The listing builds one solid part. Answer for the finished solid, in the listing's coordinates (mm). Face numbers are marked on the shaded views. A direction names the side the tool comes from. Coordinates: 2 decimals unless noted, no trailing zeros. Loops run counter-clockwise (first coordinate to the right, second up) from the corner with the lowest first, then second, coordinate; pieces in that order, holes last. Notation, with made-up numbers: (6, 72) - (13, 72) arc R18 cw to (13, 96) - close; hole circle Ø1 at (63.5, 28.5). An arc over 180 degrees is marked (long way). Write each question's results on one line, items separated by ' | '. Start each with the question number.
(1) Find section B-B on y = 14.5. Determine the outline of the cut face in (x, z) (3 decimals).
(2) Find section C-C on z = -31. Determine the outline of the cut face in (x, y) (3 decimals).
(3) For the marked faces 1 and 2, determine the directions among +Z, -Z, +X, -X, +Y, -Y from which every point of the face is accessible in a straight line to the end or side of a thin tool.
(4) Given pin 1 Ø1 at (x, y) = (-14.5, 12) entering from +Z; pin 2 Ø1.5 at (x, z) = (34.5, 5.5) entering from +Y (3 decimals); pin 3 Ø0.8 at (x, y) = (49, 13) entering from +Z (3 decimals); pin 4 Ø4.5 at (x, z) = (47.625, 57.15) entering from -Y, each flat-ended and moving along its own axis, determine where each tip first touches the part or whether it passes through.
(5) Determine the mould class of the marked faces 3, 4 and 5 for opening direction X: released by +X, released by -X, zero draft, split by the parting line, or undercut.
(6) Find section D-D on x = -26.5. Determine the outline of the cut face in (y, z) (3 decimals).
(7) Find section A-A on z = 57.15. Determine the outline of the cut face in (x, y) (3 decimals), then the cut area to 3 significant figures.
(8) Consider line 1 (X direction, y = 1.9, z = 44.45); line 2 (X direction, y = 14.75, z = 38.5); line 3 (Z direction, x = -16, y = 20.5). Determine where each line is inside the solid, lowest interval first. Write a range as from..to.
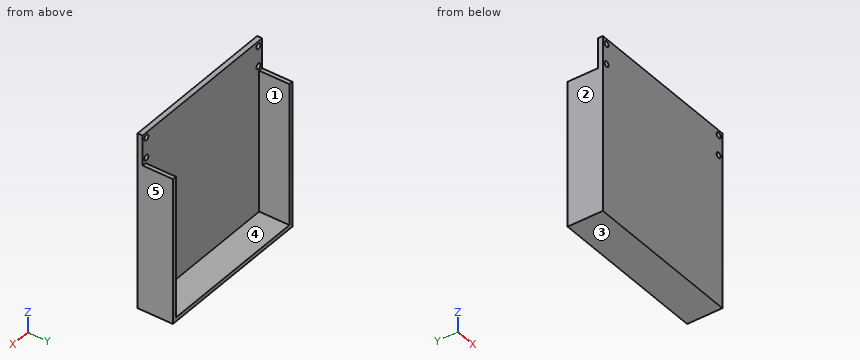
from build123d import *

# Parameters (mm, degrees)
SKETCH1_W             = 101.6
SKETCH1_H             = 101.6
SKETCH1_W_2           = 6.35
SKETCH1_H_2           = 9.525
BOSS_EXTRUDE1_DEPTH   = 3.175
F_8_32_TAPPED_HOLE1_D = 3.4544
BOSS_EXTRUDE2_DEPTH   = 19.05
SKETCH1_3_W           = 88.9
SKETCH1_3_H           = 9.525
BOSS_EXTRUDE3_DEPTH   = 3.175


with BuildPart() as part:
    # Sketch1 → Boss-Extrude1 (new body)
    with BuildSketch(Plane(origin=(0, 0, 0), x_dir=(1, 0, 0), z_dir=(0, 1, 0))):
        Rectangle(SKETCH1_W, SKETCH1_H)
        with Locations((-47.625, -55.5625)):
            Rectangle(SKETCH1_W_2, SKETCH1_H_2)
        with Locations((47.625, -55.5625)):
            Rectangle(SKETCH1_W_2, SKETCH1_H_2)
    extrude(amount=BOSS_EXTRUDE1_DEPTH)

    # #8-32 Tapped Hole1 (through all)
    with Locations(Plane(origin=(0, 0, 0), x_dir=(-1, 0, 0), z_dir=(0, -1, 0))):
        with Locations((-47.625, -57.15), (-47.625, -44.45), (47.625, -57.15), (47.625, -44.45)):
            Hole(F_8_32_TAPPED_HOLE1_D / 2)

    # Sketch8 → Boss-Extrude2 (add)
    with BuildSketch(Plane(origin=(0, 3.175, 0), x_dir=(1, 0, 0), z_dir=(0, 1, 0))):
        Polygon((-50.8, 50.8), (50.8, 50.8), (50.8, -41.275), (48.26, -41.275), (48.26, 48.26), (-48.26, 48.26), (-48.26, -41.275), (-50.8, -41.275), align=None)
    extrude(amount=BOSS_EXTRUDE2_DEPTH)

    # Sketch1<3> → Boss-Extrude3 (add)
    with BuildSketch(Plane(origin=(0, 0, 0), x_dir=(1, 0, 0), z_dir=(0, 1, 0))):
        with Locations((0, -55.5625)):
            Rectangle(SKETCH1_3_W, SKETCH1_3_H)
    extrude(amount=BOSS_EXTRUDE3_DEPTH)


solid = part.part
Values:
1) outline: (-50.8, -50.8) - (50.8, -50.8) - (50.8, 41.275) - (48.26, 41.275) - (48.26, -48.26) - (-48.26, -48.26) - (-48.26, 41.275) - (-50.8, 41.275) - close
2) outline: (-50.8, 0) - (50.8, 0) - (50.8, 22.225) - (48.26, 22.225) - (48.26, 3.175) - (-48.26, 3.175) - (-48.26, 22.225) - (-50.8, 22.225) - close
3) face 1: +Z, +Y | face 2: +Z, -Z, -X, +Y, -Y
4) pin 1: stops at z = -48.26 | pin 2: stops at y = 3.175 | pin 3: stops at z = 41.275 | pin 4: stops at y = 0
5) face 3: zero draft | face 4: undercut | face 5: released by +X
6) outline: (0, -50.8) - (22.225, -50.8) - (22.225, -48.26) - (3.175, -48.26) - (3.175, 60.325) - (0, 60.325) - close
7) outline: (-50.8, 0) - (-49.352, 0) - (-49.352, 3.175) - (-50.8, 3.175) - close; (-45.898, 0) - (45.898, 0) - (45.898, 3.175) - (-45.898, 3.175) - close; (49.352, 0) - (50.8, 0) - (50.8, 3.175) - (49.352, 3.175) - close | area: 301 mm²
8) line 1: x = -50.8..-49.35, -45.9..45.9, 49.35..50.8 | line 2: x = -50.8..-48.26, 48.26..50.8 | line 3: z = -50.8..-48.26
